Read the model definition and answer for the solid it produces. Units are mm, in the model's axes. Coordinates: 2 decimals unless noted, no trailing zeros.
(1) Straight lines are drawn through the part: line 1 along X through (y, z) = (-1.8, 100); line 2 along Z through (x, y) = (135, -2.3); line 3 along Z through (x, y) = (69, -2.75). For each, find the intervals that lie inside material, in ascending order.
(2) Determine the mould class of faces 1 (the flat face through (144, -1, 109)), 2 (the flat face through (-2, -3, -2)), 3 (the cylindrical face through (-52.068, -1.479, 43.959)) for opening direction X: pulls with the +X half, pulls with the -X half, needs draft (parallel to the pull), parting line crosses it, or undercut.
(3) The part is cut by section A-A, the plane y = -1.75. State how many separate pieces and enclosed holes the cut face has, and give its area (3 significant figures).
(4) Given pin 1 (3 mm diameter, centred on x = 135, z = -100, fed in from +Y), flat-ended and moving along its own axis, determine where the tip first touches the part or whether it passes through.
```python
from build123d import *

# Parameters (mm, degrees)
ESBO_O1_W                 = 300
ESBO_O1_H                 = 230
RESSALTO_EXTRUS_O1_DEPTH  = 3
CHANFRO1_SIZE             = 12
ESBO_O4_R                 = 8
ESBO_O4_R_2               = 7.5
CORTE_EXTRUS_O1_DEPTH     = 190.034388406
ESBO_O5_R                 = 1.75
CORTE_EXTRUS_O2_DEPTH     = 190.034388406
ESPELHAR2_COPY_1_SKETCH_R = 1.75
ESPELHAR2_COPY_1_DEPTH    = 190.034388406


with BuildPart() as part:
    # Esboço1 → Ressalto-extrusão1 (new body)
    with BuildSketch(Plane(origin=(0, 0, 0), x_dir=(1, 0, 0), z_dir=(0, 1, 0))):
        Rectangle(ESBO_O1_W, ESBO_O1_H)
    extrude(amount=-RESSALTO_EXTRUS_O1_DEPTH)

    # Chanfro1
    chanfro1_edges = [part.edges().sort_by_distance(p)[0] for p in [
        (150, -1.5, 115),
        (-150, -1.5, 115),
        (-150, -1.5, -115),
        (150, -1.5, -115),
    ]]
    chamfer(chanfro1_edges, length=CHANFRO1_SIZE)

    # Esboço4 → Corte-extrusão1 (cut, through all)
    with BuildSketch(Plane(origin=(0, 0, 0), x_dir=(1, 0, 0), z_dir=(0, 1, 0))):
        with Locations(Location((-60, -45, 0), (0, 0, 270))):
            Circle(ESBO_O4_R)
        with Locations(Location((70, -55, 0), (0, 0, 270))):
            Circle(ESBO_O4_R_2)
        with Locations(Location((70, 55, 0), (0, 0, 270))):
            Circle(ESBO_O4_R_2)
        with Locations(Location((-60, 70, 0), (0, 0, 270))):
            Circle(ESBO_O4_R_2)
        with BuildLine():
            Line((-62.5, -21.75), (-57.5, -21.75))
            ThreePointArc((-57.5, -21.75), (-55.75, -20), (-57.5, -18.25))
            Line((-57.5, -18.25), (-62.5, -18.25))
            ThreePointArc((-62.5, -18.25), (-64.25, -20), (-62.5, -21.75))
        make_face()
        with BuildLine():
            Line((-38.614909362, -54.459936491), (-41.114909362, -58.790063509))
            ThreePointArc((-41.114909362, -58.790063509), (-40.474364905, -61.180607966), (-38.083820449, -60.540063509))
            Line((-38.083820449, -60.540063509), (-35.583820449, -56.209936491))
            ThreePointArc((-35.583820449, -56.209936491), (-36.224364905, -53.819392034), (-38.614909362, -54.459936491))
        make_face()
        with BuildLine():
            Line((-78.885090638, -58.790063509), (-81.385090638, -54.459936491))
            ThreePointArc((-81.385090638, -54.459936491), (-83.775635095, -53.819392034), (-84.416179551, -56.209936491))
            Line((-84.416179551, -56.209936491), (-81.916179551, -60.540063509))
            ThreePointArc((-81.916179551, -60.540063509), (-79.525635095, -61.180607966), (-78.885090638, -58.790063509))
        make_face()
        with BuildLine():
            Line((67.5, -28.25), (72.5, -28.25))
            ThreePointArc((72.5, -28.25), (74.25, -30), (72.5, -31.75))
            Line((72.5, -31.75), (67.5, -31.75))
            ThreePointArc((67.5, -31.75), (65.75, -30), (67.5, -28.25))
        make_face()
        with BuildLine():
            Line((91.385090638, -64.459936491), (88.885090638, -68.790063509))
            ThreePointArc((88.885090638, -68.790063509), (89.525635095, -71.180607966), (91.916179551, -70.540063509))
            Line((91.916179551, -70.540063509), (94.416179551, -66.209936491))
            ThreePointArc((94.416179551, -66.209936491), (93.775635095, -63.819392034), (91.385090638, -64.459936491))
        make_face()
        with BuildLine():
            Line((51.114909362, -68.790063509), (48.614909362, -64.459936491))
            ThreePointArc((48.614909362, -64.459936491), (46.224364905, -63.819392034), (45.583820449, -66.209936491))
            Line((45.583820449, -66.209936491), (48.083820449, -70.540063509))
            ThreePointArc((48.083820449, -70.540063509), (50.474364905, -71.180607966), (51.114909362, -68.790063509))
        make_face()
        with BuildLine():
            Line((67.5, 81.75), (72.5, 81.75))
            ThreePointArc((72.5, 81.75), (74.25, 80), (72.5, 78.25))
            Line((72.5, 78.25), (67.5, 78.25))
            ThreePointArc((67.5, 78.25), (65.75, 80), (67.5, 81.75))
        make_face()
        with BuildLine():
            Line((91.385090638, 45.540063509), (88.885090638, 41.209936491))
            ThreePointArc((88.885090638, 41.209936491), (89.525635095, 38.819392034), (91.916179551, 39.459936491))
            Line((91.916179551, 39.459936491), (94.416179551, 43.790063509))
            ThreePointArc((94.416179551, 43.790063509), (93.775635095, 46.180607966), (91.385090638, 45.540063509))
        make_face()
        with BuildLine():
            Line((51.114909362, 41.209936491), (48.614909362, 45.540063509))
            ThreePointArc((48.614909362, 45.540063509), (46.224364905, 46.180607966), (45.583820449, 43.790063509))
            Line((45.583820449, 43.790063509), (48.083820449, 39.459936491))
            ThreePointArc((48.083820449, 39.459936491), (50.474364905, 38.819392034), (51.114909362, 41.209936491))
        make_face()
        with BuildLine():
            Line((-62.5, 86.75), (-57.5, 86.75))
            ThreePointArc((-57.5, 86.75), (-55.75, 88.5), (-57.5, 90.25))
            Line((-57.5, 90.25), (-62.5, 90.25))
            ThreePointArc((-62.5, 90.25), (-64.25, 88.5), (-62.5, 86.75))
        make_face()
        with BuildLine():
            Line((-43.25, 72.5), (-43.25, 67.5))
            ThreePointArc((-43.25, 67.5), (-41.5, 65.75), (-39.75, 67.5))
            Line((-39.75, 67.5), (-39.75, 72.5))
            ThreePointArc((-39.75, 72.5), (-41.5, 74.25), (-43.25, 72.5))
        make_face()
        with BuildLine():
            Line((-57.5, 53.25), (-62.5, 53.25))
            ThreePointArc((-62.5, 53.25), (-64.25, 51.5), (-62.5, 49.75))
            Line((-62.5, 49.75), (-57.5, 49.75))
            ThreePointArc((-57.5, 49.75), (-55.75, 51.5), (-57.5, 53.25))
        make_face()
        with BuildLine():
            Line((-76.75, 67.5), (-76.75, 72.5))
            ThreePointArc((-76.75, 72.5), (-78.5, 74.25), (-80.25, 72.5))
            Line((-80.25, 72.5), (-80.25, 67.5))
            ThreePointArc((-80.25, 67.5), (-78.5, 65.75), (-76.75, 67.5))
        make_face()
    extrude(amount=-CORTE_EXTRUS_O1_DEPTH, mode=Mode.SUBTRACT)

    # Esboço5 → Corte-extrusão2 (cut, through all)
    with BuildSketch(Plane(origin=(0, 0, 0), x_dir=(1, 0, 0), z_dir=(0, 1, 0))):
        with Locations(Location((-135, -100, 0), (0, 0, 270))):
            Circle(ESBO_O5_R)
    corte_extrus_o2 = extrude(amount=-CORTE_EXTRUS_O2_DEPTH, mode=Mode.SUBTRACT)

    # Espelhar1: Corte-extrusão2 across plane
    add(corte_extrus_o2.mirror(Plane.XY), mode=Mode.SUBTRACT)

    # Espelhar2: Corte-extrusão2 across plane
    add(corte_extrus_o2.mirror(Plane(origin=(0, 0, 0), x_dir=(0, 0, 1), z_dir=(1, 0, 0))), mode=Mode.SUBTRACT)

    # Espelhar2 copy 1 sketch → Espelhar2 copy 1 (cut, through all)
    with BuildSketch(Plane(origin=(0, 0, 0), x_dir=(-1, 0, 0), z_dir=(0, 1, 0))):
        with Locations(Location((-135, -100, 0), (0, 0, 270))):
            Circle(ESPELHAR2_COPY_1_SKETCH_R)
    extrude(amount=-ESPELHAR2_COPY_1_DEPTH, mode=Mode.SUBTRACT)


solid = part.part
```
Computed:
1. line 1: x = -150 to -136.75, -133.25 to 133.25, 136.75 to 150
1. line 2: z = -115 to -101.75, -98.25 to 98.25, 101.75 to 115
1. line 3: z = -115 to -81.75, -78.25 to -62.43, -47.57 to 28.25, 31.75 to 47.57, 62.43 to 115
2. face 1: pulls with the +X half
2. face 2: needs draft
2. face 3: undercut
3. separate pieces: 1
3. enclosed holes: 21
3. area: 67,600 mm2
4. pin 1: passes through
